Source: CAD feature listing. Evaluate the final solid. Frame: model axes, mm. A direction names the side the tool comes from. Give positions to 0.01 mm unless a question says otherwise; leave off trailing zeros. Loops run counter-clockwise (first coordinate to the right, second up) from the corner with the lowest first, then second, coordinate; pieces in that order, holes last. Notation, with made-up numbers: M 70,-3.75 L 120,-3.75 A23 cw 120,32.25 Z; hole C 31.5,-22 d6. An arc over 180 degrees is marked long. Put each result on its own line as item: value.
from build123d import *

# Parameters (mm, degrees)
F1_DEPTH = 25
F2_T     = -2.5
F3_R     = 8.0738328397
F4_DEPTH = 25


with BuildPart() as f1:
    # F0 (on Front) → F1 (new body)
    with BuildSketch(Plane.XZ):
        with BuildLine():
            ThreePointArc((-102.7760443896, -106.6724830235), (49.3553380224, -110.5098127391), (201.5178711407, -108.2193697847))
            ThreePointArc((201.5178711407, -108.2193697847), (213.1602276304, -26.1415825476), (189.002040682, 53.1596761167))
            ThreePointArc((189.002040682, 53.1596761167), (72.260836705, 55.8025234443), (-44.4803672719, 53.1596761167))
            ThreePointArc((-44.4803672719, 53.1596761167), (-97.433719622, 49.5356960569), (-102.7760443896, -3.2719768957))
            ThreePointArc((-102.7760443896, -3.2719768957), (-107.2862833974, -54.9722299596), (-102.7760443896, -106.6724830235))
        make_face()
        Polygon((58.9537048383, -18.80859987), (77.1279207266, -4.826139813), (98.3241942876, -13.5742424376), (101.3462519602, -36.3048051192), (83.1720360719, -50.2872651763), (61.975762511, -41.5391625517), align=None, mode=Mode.SUBTRACT)
    extrude(amount=F1_DEPTH)

    # F2
    f2_openings = [f1.faces().sort_by_distance(p)[0] for p in [
        (49.796749, -25, -27.587864),
    ]]
    offset(amount=F2_T, openings=f2_openings, kind=Kind.INTERSECTION)

    # F3 (on face) → F4 (join)
    with BuildSketch(Plane.XZ.offset(2.5)):
        with Locations((-36.8073508143, -34.8820904728)):
            Circle(F3_R)
    extrude(amount=F4_DEPTH)


solid = f1.part
1. Section query B-B (x = -53). Output: boundary loops of the cut face in (y, z), plus the area to 3 significant figures.
Found:
outline: M -25,-108.6 L 0,-108.6 L 0,57.96 L -25,57.96 L -25,55.24 L -2.5,55.24 L -2.5,-106.1 L -25,-106.1 Z
area: 534 mm^2
2. Contact query for flat-ended pins moving along their axis: P1, Ø6, axis at x = 170, z = 13, coming from the -Y side; P2, Ø1.5, axis at x = 145, y = -12, coming from the -Z side; P3, Ø4, axis at x = 119.5, y = -8.5, coming from the +Z side; P4, Ø1, axis at x = -38, z = -51, coming from the +Y side. Output: stop coordinate, or through.
Found:
P1: y = -2.5
P2: z = -109.8
P3: z = 55.41
P4: y = 0
3. Access query for faces 5 (the flat face through (66.37, -13.59, -9.95)), 6 (the flat face through (72.722, -12.325, -45.974)), 7 (the flat face through (-37, -27.5, -35)). Directions: +Z, -Z, +X, -X, +Y, -Y. A direction counts if a zero-diameter tool reaches every point of the face in a straight line with its end or side. Return the directions, or none.
Found:
face 5: -Y
face 6: +Y, -Y
face 7: +Z, -Z, +X, -X, -Y
4. Draft query along Z for faces 1 (the cylindrical face through (-42.76, -14.82, -29.43)), 2 (the cylindrical face through (47.2, -12.3, -110.5)), 3 (the cylindrical face through (73.896, -12.325, 55.802)), 4 (the flat face through (50, 0, -24)). Return one class per face: pulls with the +Z half, pulls with the -Z half, needs draft (parallel to the pull), parting line crosses it, or undercut.
Found:
face 1: undercut
face 2: pulls with the -Z half
face 3: pulls with the +Z half
face 4: needs draft
5. Section query C-C (z = 9). Output: boundary loops of the cut face in (x, y), plus the area to 3 significant figures.
Found:
outline: M -108.48,-25 L -105.88,-25 L -105.88,-2.5 L 204.51,-2.5 L 204.51,-25 L 207.1,-25 L 207.1,0 L -108.48,0 Z
area: 906 mm^2
6. Section query A-A (y = -19.75). Output: boundary loops of the cut face in (x, z), plus the area to 3 significant figures.
Found:
outline: M -102.78,-106.67 A3779.25 ccw 201.52,-108.22 A191.39 ccw 189,53.16 A2579.7 ccw -44.48,53.16 A41.15 ccw -102.78,-3.27 A298.57 ccw Z; C -36.81,-34.88 d16.15; M 56.29,-17.71 L 59.69,-43.3 L 83.55,-53.15 L 104.01,-37.41 L 100.61,-11.81 L 76.75,-1.96 Z; hole M -100.65,-104.27 A3776.75 ccw 199.76,-105.78 A188.89 ccw 187.5,50.72 A2577.2 ccw -45.26,50.62 A38.65 ccw -100.13,-2.68 A296.07 ccw Z; hole M 58.95,-18.81 L 61.98,-41.54 L 83.17,-50.29 L 101.35,-36.3 L 98.32,-13.57 L 77.13,-4.83 Z
area: 2,860 mm^2
7. Material intervals for line 1 (Z direction, x = 71, y = -14.25); line 2 (X direction, y = -9.75, z = -23); line 3 (Z direction, x = 72, y = -12.75), sorted ascending. Write a range as from..to.
Found:
line 1: -110.56..-108.06, -47.97..-45.26, -9.54..-6.39, 53.3..55.8
line 2: -105.57..-103.05, 56.99..59.51, 99.58..102.1, 210.38..212.89
line 3: -110.56..-108.06, -48.38..-45.68, -8.77..-5.62, 53.3..55.8
